The drawing under review shows one solid part. Ordinate dimensions are in mm from its lowest x, y, z. A direction names the side the tool comes from. Coordinates: 2 decimals unless noted, no trailing zeros. Loops run counter-clockwise (first coordinate to the right, second up) from the corner with the lowest first, then second, coordinate; pieces in that order, holes last. Notation, with made-up numbers: M 16,34.5 L 75,34.5 A29 ccw 75,69.5 Z; hole C 14.25,17 d4. An arc over 180 degrees is marked long. Put each result on its own line as item: value.
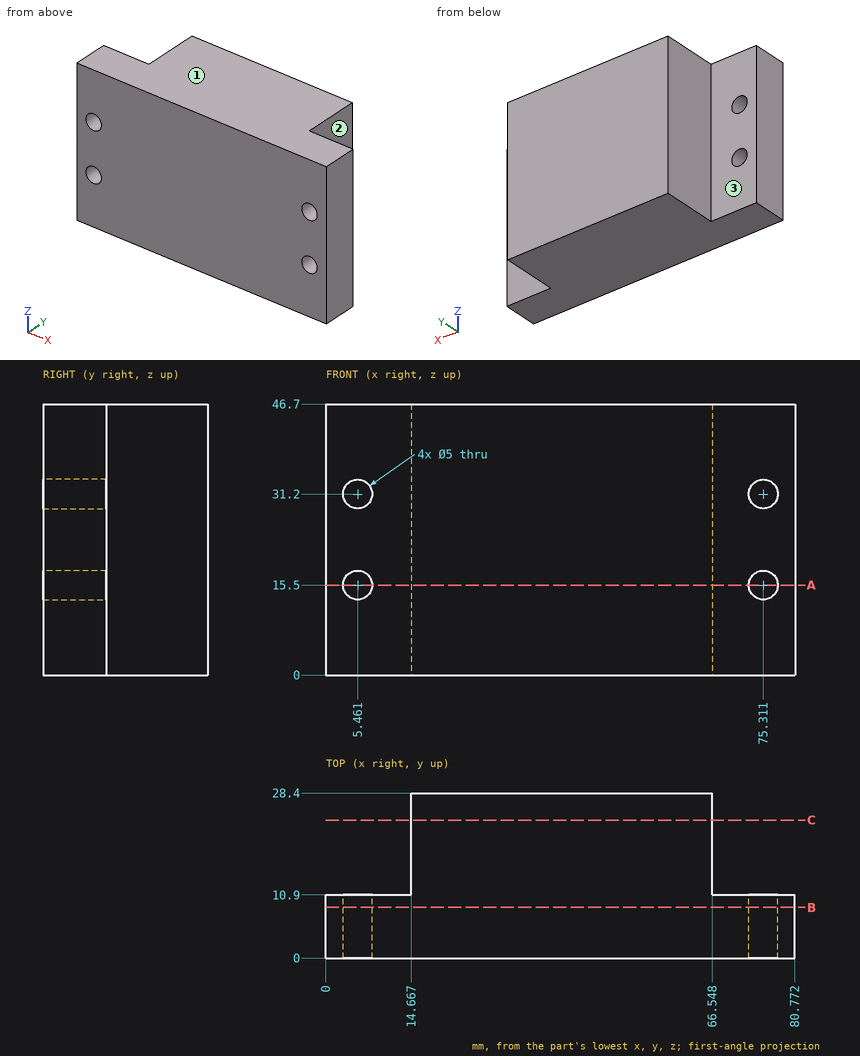
(1) Wall thickness on line 1 along X through (y, z) = (8, 15.5); line 2 along Z through (x, y) = (74.5, 6.25) (1 decimal); line 3 along Y through (x, z) = (71, 15): over which ranges is each line inside the solid? List them lowest first. Write a range as [from, to].
Determined:
line 1: x = [0, 2.96], [7.96, 72.81], [77.81, 80.77]
line 2: z = [0, 13.1], [17.9, 28.8], [33.6, 46.7]
line 3: y = [0, 10.9]
(2) Tool access review of the marked faces 1, 2 and 3: name each direction out of +Z, -Z, +X, -X, +Y, -Y from which nothing blocks a thin tool from reaching the whole face with its end or side.
Determined:
face 1: +Z, +X, -X, +Y, -Y
face 2: +Z, -Z, +X, +Y
face 3: +Z, -Z, -X, +Y
(3) Add section B-B (y = 8.75). Write out the cut boundary in (x, z).
Determined:
outline: M 0,0 L 80.77,0 L 80.77,46.7 L 0,46.7 Z; hole C 5.46,15.5 d5; hole C 5.46,31.2 d5; hole C 75.31,15.5 d5; hole C 75.31,31.2 d5
(4) For pin 1 (5 mm diameter, centred on x = 69.5, z = 20, fed in from -Y); pin 2 (4 mm diameter, centred on x = 5.461, z = 31.2, fed in from +Y); pin 3 (7.5 mm diameter, centred on x = 9.5, z = 23.5, fed in from +Y), all flat-tipped, find the tip position at first contact; note any pin that passes through.
Determined:
pin 1: stops at y = 0
pin 2: passes through
pin 3: stops at y = 10.9
(5) Add section A-A (z = 15.5). Write out the cut boundary in (x, y), plus the area to 3 significant figures.
Determined:
outline: M 0,0 L 2.96,0 L 2.96,10.9 L 0,10.9 Z; M 7.96,0 L 72.81,0 L 72.81,10.9 L 66.55,10.9 L 66.55,28.4 L 14.67,28.4 L 14.67,10.9 L 7.96,10.9 Z; M 77.81,0 L 80.77,0 L 80.77,10.9 L 77.81,10.9 Z
area: 1,680 mm^2
(6) Add section C-C (y = 23.75). Write out the cut boundary in (x, z).
Determined:
outline: M 14.67,0 L 66.55,0 L 66.55,46.7 L 14.67,46.7 Z
